Could you check a few things on this model? Use its own coordinates, in mm. A direction names the side the tool comes from. Give positions to 0.01 mm unless a question says otherwise; leave off trailing zeros. Loops run counter-clockwise (first coordinate to the right, second up) from the corner with the lowest first, then second, coordinate; pieces in that order, holes last. Notation, with made-up numbers: (-35, 53) - (-24, 53) arc R18 ccw to (-24, 69) - close; hole circle Ø3 at (-3.5, 59). An arc over 180 degrees is marked (long way). Write each question's results on one line, items separated by ' | '. Start each with the question number.
1) I want a section at C-C, the plane x = 7.5. Write out the boundary of the cut face in (y, z), and give its area (3 significant figures).
2) I'm going to push flat-ended pins straight in: pin 1 (4 mm diameter, centred on x = -15.5, z = -2, fed in from -Y); pin 2 (3.5 mm diameter, centred on x = 19, y = -21, fed in from -Z); pin 3 (6.5 mm diameter, centred on x = -21, y = -13, fed in from -Z); pin 4 (2 mm diameter, centred on x = 17.5, z = 2.5, fed in from -Y). Where does each tip first touch, or does it pass through?
3) I want a section at D-D, the plane z = 4.75. Write out the boundary of the cut face in (x, y).
4) If I drill on probe 1 along Y at (x, z) = (0, -6.8); probe 2 along Z at (x, y) = (21.5, 21); probe 3 along Z at (x, y) = (7, 5.5), over which ranges is the centre line in solid material (lowest first)? Write a range as [from, to].
5) On a 3-axis mill with a long thin cutter (end or side, diameter ignored), from which of +Z, -Z, +X, -X, +Y, -Y can I reach the whole of each face in a straight line? I mean faces 4 (the face through (22.4, 0.1, -1.25)), 5 (the face through (19, 18, -6.75)), 6 (the face through (22, 4.375, 0)), 7 (the face through (-21.97, 20.01, -0.39)). Say none if no direction works.
6) If we mould it in two halves opening along Y, with no side actions, what happens to faces 1 (the face through (17.587, -13.813, -0.395)), 2 (the face through (-22.2, -11.3, -1.25)), 3 (the face through (-16.76, 24.53, -0.39))? For each: +Y half, -Y half, draft (parallel to the pull), parting line (faces both ways), or undercut.
7) I want a section at B-B, the plane y = 0. Write out the boundary of the cut face in (x, z).
8) I want a section at A-A, the plane x = 19. Write out the boundary of the cut face in (y, z).
from build123d import *

# Parameters (mm, degrees)
F0_R          = 2.25
F1_DEPTH      = 7
F1_DEPTH_BACK = 8
F2_R          = 16
F3_DEPTH      = 3
F4_W          = 12
F4_H          = 2.605645
F4_W_2        = 2.164235
F4_H_2        = 8.75
F5_DEPTH      = 1.25
F6_W          = 17
F6_H          = 12.5
F7_DEPTH      = 15


with BuildPart() as f1:
    # F0 (on Top) → F1 (new body, two sides)
    with BuildSketch(Plane.XY) as f1_sk:
        with BuildLine():
            Line((26, 8), (26, 27.5))
            Line((26, 27.5), (0, 27.5))
            ThreePointArc((0, 27.5), (-7.390942, 26.488186), (-14.23801, 23.527198))
            ThreePointArc((-14.23801, 23.527198), (-15.246821, 23.32858), (-16.146537, 23.826232))
            Line((-16.146537, 23.826232), (-17.396611, 25.263817))
            ThreePointArc((-17.396611, 25.263817), (-22.263817, 25.603389), (-22.603389, 20.736183))
            Line((-22.603389, 20.736183), (-21.316096, 19.255796))
            ThreePointArc((-21.316096, 19.255796), (-20.949135, 18.329769), (-21.243133, 17.378059))
            ThreePointArc((-21.243133, 17.378059), (-19.890092, -13.900871), (10.993048, -19.042257))
            ThreePointArc((10.993048, -19.042257), (11.971845, -18.865751), (12.845895, -19.340339))
            Line((12.845895, -19.340339), (16.441702, -23.314651))
            ThreePointArc((16.441702, -23.314651), (21.314651, -23.558298), (21.558298, -18.685349))
            Line((21.558298, -18.685349), (17.971026, -14.720469))
            ThreePointArc((17.971026, -14.720469), (17.585694, -13.798288), (17.865245, -12.838731))
            ThreePointArc((17.865245, -12.838731), (21.677485, -3.753219), (21.1417, 6.085106))
            ThreePointArc((21.1417, 6.085106), (21.384776, 7.402125), (22.58318, 8))
            Line((22.58318, 8), (26, 8))
        make_face()
        with Locations((19, -21)):
            Circle(F0_R, mode=Mode.SUBTRACT)
        with Locations((-20, 23)):
            Circle(F0_R, mode=Mode.SUBTRACT)
    extrude(amount=F1_DEPTH)
    extrude(f1_sk.sketch, amount=-F1_DEPTH_BACK)

    # F2 (on face) → F3 (cut)
    with BuildSketch(Plane(origin=(0, 0, -8), x_dir=(1, 0, 0), z_dir=(0, 0, -1))):
        Circle(F2_R)
    extrude(amount=-F3_DEPTH, mode=Mode.SUBTRACT)

    # F4 (on Top) → F5 (join, symmetric)
    with BuildSketch(Plane.XY):
        with Locations((20, 27.097178)):
            Rectangle(F4_W, F4_H)
        with Locations((21.917882, 0)):
            Rectangle(F4_W_2, F4_H_2)
        Polygon((-22.531997, -6.254788), (-25.167336, -8), (-20.336118, -15.29533), (-17.700779, -13.550117), align=None)
    extrude(amount=F5_DEPTH, both=True)

    # F6 (on face) → F7 (cut)
    with BuildSketch(Plane.YZ.offset(26)):
        with Locations((17.75, -0.5)):
            Rectangle(F6_W, F6_H)
    extrude(amount=-F7_DEPTH, mode=Mode.SUBTRACT)


solid = f1.part
Answers:
1) outline: (-20.68, -8) - (-14.13, -8) - (-14.13, -5) - (14.13, -5) - (14.13, -8) - (27.5, -8) - (27.5, 7) - (-20.68, 7) - close | area: 638 mm2
2) pin 1: stops at y = -19.07 | pin 2: passes through | pin 3: stops at z = -8 | pin 4: stops at y = -24.41
3) outline: (-22.6, 20.74) - (-21.32, 19.26) arc R1.5 cw to (-21.24, 17.38) arc R24.86 ccw to (10.99, -19.04) arc R1.5 cw to (12.85, -19.34) - (16.44, -23.31) arc R3.45 ccw to (21.56, -18.69) - (17.97, -14.72) arc R1.5 cw to (17.87, -12.84) arc R22 ccw to (21.14, 6.09) arc R1.5 cw to (22.58, 8) - (26, 8) - (26, 9.25) - (11, 9.25) - (11, 26.25) - (26, 26.25) - (26, 27.5) - (0, 27.5) arc R27.5 ccw to (-14.24, 23.53) arc R1.5 cw to (-16.15, 23.83) - (-17.4, 25.26) arc R3.45 ccw to start; hole circle Ø4.5 at (-20, 23); hole circle Ø4.5 at (19, -21)
4) probe 1: y = [-22.25, -16], [16, 27.5] | probe 2: z = [-8, -6.75], [5.75, 7] | probe 3: z = [-5, 7]
5) face 4: -Z, +X | face 5: +X | face 6: +Z, -Z, +X | face 7: +Z, -Z, -X
6) face 1: undercut | face 2: draft | face 3: +Y half
7) outline: (-26, -8) - (-16, -8) - (-16, -5) - (16, -5) - (16, -8) - (22, -8) - (22, -1.25) - (23, -1.25) - (23, 1.25) - (22, 1.25) - (22, 7) - (-26, 7) - close
8) outline: (-24.45, -8) - (-23.25, -8) - (-23.25, 7) - (-24.45, 7) - close; (-18.75, -8) - (-15.86, -8) - (-15.86, 7) - (-18.75, 7) - close; (-11.09, -8) - (27.5, -8) - (27.5, -1.25) - (28.4, -1.25) - (28.4, 1.25) - (27.5, 1.25) - (27.5, 7) - (-11.09, 7) - close; hole (9.25, -6.75) - (26.25, -6.75) - (26.25, 5.75) - (9.25, 5.75) - close
